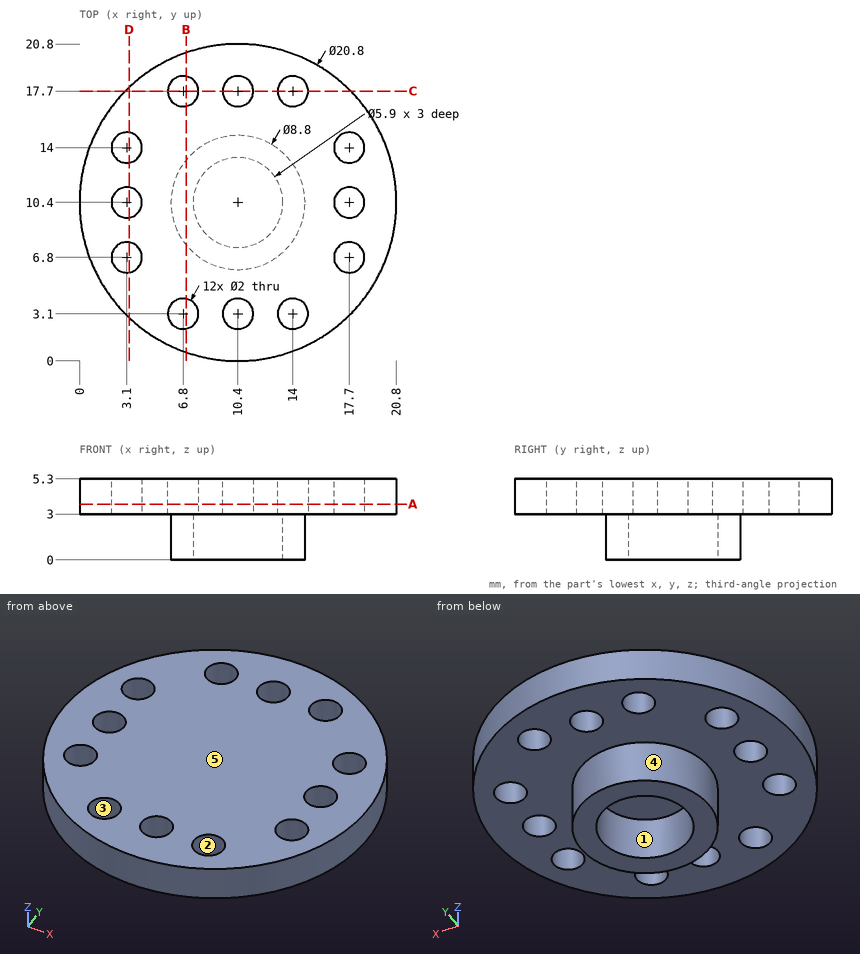
For this review, use the dimensioned drawing (mm, ordinates from the lowest corner) and the shaded views. A direction names the side the tool comes from. Give positions to 0.01 mm unless a question says otherwise; leave off trailing zeros. Loops run counter-clockwise (first coordinate to the right, second up) from the corner with the lowest first, then second, coordinate; pieces in that order, holes last.
Item 1: For line 1 along Y through (x, z) = (10.4, 4.65); line 2 along Y through (x, z) = (7.5, 3.95); line 3 along Z through (x, y) = (4, 11.5), list the stretches that pass through material, from the lowest coordinate up.
Item 2: Insertion check: pin 1 (1.6 mm diameter, centred on x = 14, y = 17.7, fed in from -Z); pin 2 (5 mm diameter, centred on x = 18.5, y = 8.5, fed in from -Z). Each pin has a flat end and moves straight along its axis. Give the tip position at first contact, or say it passes through.
Item 3: Tool access review of the marked faces 1 and 2: name each direction out of +Z, -Z, +X, -X, +Y, -Y from which nothing blocks a thin tool from reaching the whole face with its end or side.
Item 4: Take a section at D-D, the plane x = 3.25. State the section outline as (y, z) points.
Item 5: Take a section at C-C, the plane y = 17.7. State the section outline as (x, z) points, and give its area (3 significant figures).
Item 6: Take a section at B-B, the plane x = 7. State the section outline as (y, z) points.
Item 7: Draft analysis for pull direction Y (two halves, no side actions). For the marked faces 3, 4 and 5, state which applies: +Y half, -Y half, draft (parallel to the pull), parting line (faces both ways), or undercut.
Item 8: Take a section at A-A, the plane z = 3.65. Give the number of separate pieces and of enclosed holes in the cut face, and give its area (3 significant figures).
Calculated:
1. line 1: y = 0 to 2.1, 4.1 to 16.7, 18.7 to 20.8
1. line 2: y = 0.41 to 2.39, 3.81 to 16.99, 18.41 to 20.39
1. line 3: z = 3 to 5.3
2. pin 1: passes through
2. pin 2: stops at z = 3
3. face 1: -Z
3. face 2: +Z, -Z
4. outline: (2.85, 3) - (5.81, 3) - (5.81, 5.3) - (2.85, 5.3) - close; (7.79, 3) - (9.41, 3) - (9.41, 5.3) - (7.79, 5.3) - close; (11.39, 3) - (13.01, 3) - (13.01, 5.3) - (11.39, 5.3) - close; (14.99, 3) - (17.95, 3) - (17.95, 5.3) - (14.99, 5.3) - close
5. outline: (2.99, 3) - (5.8, 3) - (5.8, 5.3) - (2.99, 5.3) - close; (7.8, 3) - (9.4, 3) - (9.4, 5.3) - (7.8, 5.3) - close; (11.4, 3) - (13, 3) - (13, 5.3) - (11.4, 5.3) - close; (15, 3) - (17.81, 3) - (17.81, 5.3) - (15, 5.3) - close
5. area: 20.3 mm2
6. outline: (0.57, 3) - (2.12, 3) - (2.12, 5.3) - (0.57, 5.3) - close; (4.08, 3) - (7.61, 3) - (7.61, 0) - (13.19, 0) - (13.19, 3) - (16.72, 3) - (16.72, 5.3) - (4.08, 5.3) - close; (18.68, 3) - (20.23, 3) - (20.23, 5.3) - (18.68, 5.3) - close
7. face 3: undercut
7. face 4: parting line
7. face 5: draft
8. separate pieces: 1
8. enclosed holes: 12
8. area: 302 mm2
